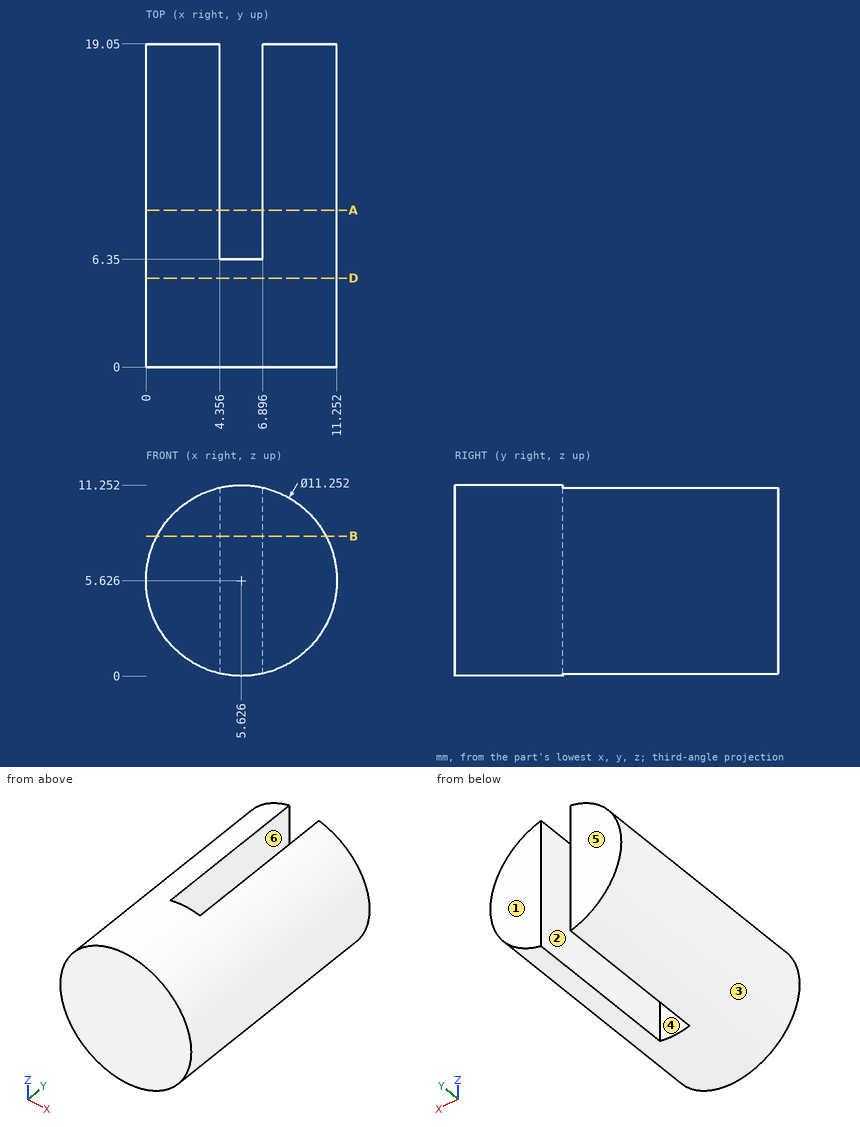
Could you check a few things on this drawing? It's one solid part, dimensions in mm from its lowest x, y, z. A direction names the side the tool comes from. Give positions to 0.01 mm unless a question says otherwise; leave off trailing zeros. Order: outer loops, then holes, each group sorted by start corner. A loop starts at its lowest first (then second) coordinate and runs counter-clockwise, first axis right, second up. Notation, with made-up numbers: (69.5, 81) - (99.5, 81) arc R20 ccw to (99.5, 105) - close; hole circle Ø3 at (64.5, -17.5). An arc over 180 degrees is marked (long way). Answer as a JSON object with one key per item and string values. Group by question number.
Item 1: If we section it at D-D on y = 5.25: Please give me the cut outline in (x, z).
Item 2: If we mould it in two halves opening along X, with no side actions, what happens to the marked faces 1, 2, 3 and 4? For each: pulls with the +X half, pulls with the -X half, needs draft (parallel to the pull), parting line crosses it, or undercut.
Item 3: Which directions (+Z, -Z, +X, -X, +Y, -Y) give clear straight access to the entire face, cutting with the end or side of a thin tool? Please do the marked faces 5 and 6.
Item 4: If we section it at B-B on z = 8.25: Please give me the cut outline in (x, y), and give its area (3 significant figures).
Item 5: For P1, Ø2, axis at x = 3, y = 8.5, coming from the -Z side; P2, Ø5, axis at x = 3.5, y = 8, coming from the -Z side; P3, Ø1, axis at y = 6.5, z = 4.5, coming from the +X side; P4, Ø1.5, axis at x = 6, y = 7.5, coming from the +Z side, each with a flat end and sliding along its axis, tell me the tip position at first contact or that it passes through.
Item 6: Please list where these lines run through material, in increasing order: probe 1 along Y at (x, z) = (5, 6); probe 2 along X at (y, z) = (15.25, 9.75) (1 decimal).
Item 7: If we section it at A-A on y = 9.25: Please give me the cut outline in (x, z) (1 decimal).
Result set:
{
 "1": {"outline": "circle Ø11.25 at (5.63, 5.63)"},
 "2": {"face 1": "needs draft", "face 2": "undercut", "face 3": "parting line crosses it", "face 4": "undercut"},
 "3": {"face 5": "+Z, -Z, +X, -X, +Y", "face 6": "+Z, -Z, +Y"},
 "4": {"outline": "(0.65, 0) - (10.6, 0) - (10.6, 19.05) - (6.9, 19.05) - (6.9, 6.35) - (4.36, 6.35) - (4.36, 19.05) - (0.65, 19.05) - close", "area": "157 mm²"},
 "5": {"P1": "z = 0.24", "P2": "z = 0.01", "P3": "x = 11.22", "P4": "through"},
 "6": {"probe 1": "0 to 6.35", "probe 2": "1.8 to 4.4, 6.9 to 9.5"},
 "7": {"outline": "(4.4, 0.1) - (4.4, 11.1) arc R5.6 ccw to start; (6.9, 0.1) arc R5.6 ccw to (6.9, 11.1) - close"}
}
